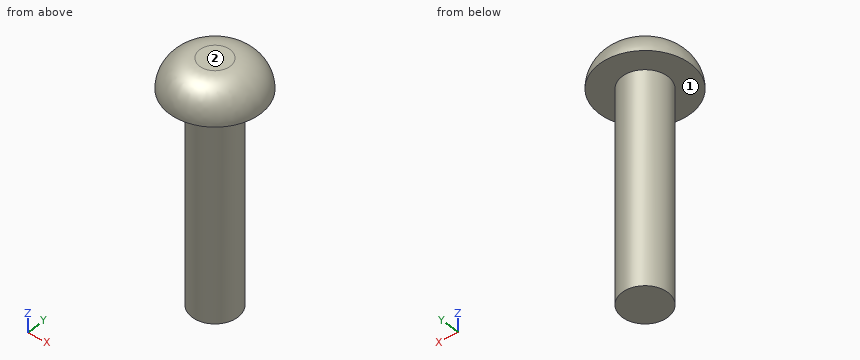
Autodesk Inventor part; units mm, degrees
ref_plane "YZ Plane" through (0, 0, 0) normal (1, 0, 0) x (0, 1, 0)
ref_plane "XZ Plane" through (0, 0, 0) normal (0, 1, 0) x (-1, 0, 0)
ref_plane "XY Plane" through (0, 0, 0) normal (0, 0, 1) x (1, 0, 0)
sketch "スケッチ1" plane through (0, 0, 0) normal (0, 0, 1) x (1, 0, 0)
  circle A0 centre (0, 0) radius 1.5
  dimension "d0" = 3
extrude "押し出し1" add sketch "スケッチ1" along normal blind 14
sketch "スケッチ2" plane through (0, 0, 14) normal (0, 0, 1) x (1, 0, 0)
  circle A0 centre (0, 0) radius 1.5
  circle A1 centre (0, 0) radius 3
  dimension "d3" = 6
extrude "押し出し2" add sketch "スケッチ2" along normal blind 2 contours A0 | A1
fillet "フィレット1" radius 2 1 edges at (-3, 0, 16)
properties part number "M3ボタンボルト14" material "鋼、高強度、低合金"
The listing builds one solid part. Answer for the finished solid, in the listing's coordinates (mm). Face numbers are marked on the shaded views. A direction names the side the tool comes from. Give positions to 0.01 mm unless a question says otherwise; leave off trailing zeros. Order: outer loops, then holes, each group sorted by start corner. A loop starts at its lowest first (then second) coordinate and runs counter-clockwise, first axis right, second up. Notation, with made-up numbers: (61, -17.5) -> (84, -17.5) arc R29 cw to (84, 18.5) -> close; hole circle Ø4 at (15.5, -36.5). An arc over 180 degrees is marked (long way). One line per item, written item: value.
1) Flat-ended cylindrical pins translate along their axes: P1, Ø3, axis at x = 2, y = -1.5, coming from the -Z side; P2, Ø1.5, axis at x = -1.5, z = 10.5, coming from the +Y side; P3, Ø1.5, axis at x = -1.5, z = 10, coming from the -Y side. Find the tip coordinate at first contact, or state that the pin passes through.
Reported:
P1: stops at z = 0
P2: stops at y = 1.3
P3: stops at y = -1.3
2) Find the intervals of material crossed by line 1 (Z direction, x = -1, y = 0.5); line 2 (Y direction, x = -0.5, z = 3); line 3 (Y direction, x = 1, z = 4), in increasing order.
Reported:
line 1: z = 0 to 16
line 2: y = -1.41 to 1.41
line 3: y = -1.12 to 1.12
3) A tool of negligible diameter and unlimited length cuts with its end or side. For the marked faces 1 and 2, from which of +Z, -Z, +X, -X, +Y, -Y can it reach the whole face along a straight path? Write none if from no direction.
Reported:
face 1: -Z
face 2: +Z, +X, -X, +Y, -Y
4) Find section A-A, the plane z = 13.75. Determine the outline of the cut face in (x, y), plus the area to 3 significant figures.
Reported:
outline: circle Ø3 at (0, 0)
area: 7.07 mm^2
